Input: dimensioned drawing with shaded views. Units: mm. Origin: part minimum x, y, z. Give positions to 0.01 mm unless a question says otherwise; leave off trailing zeros. Order: outer loops, then holes, each group sorted by start corner. A loop starts at its lowest first (then second) coordinate and runs counter-clockwise, first axis right, second up.
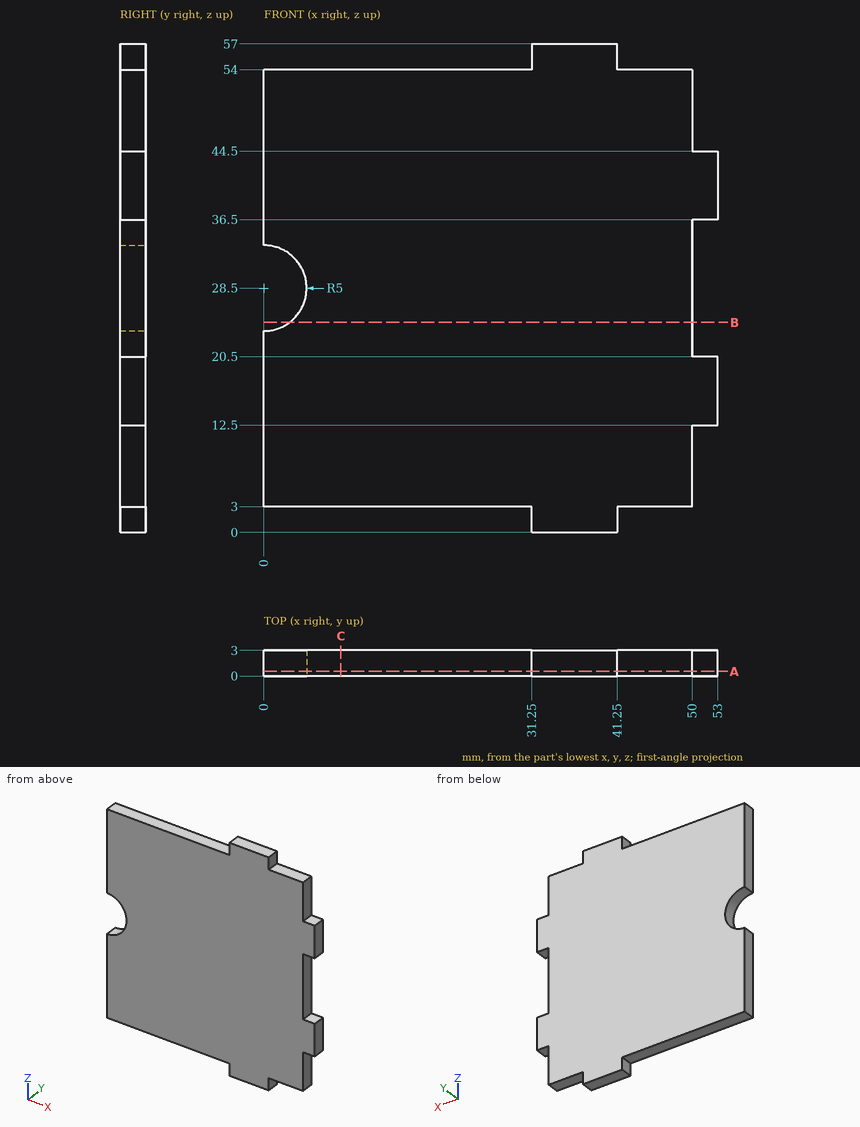
1) Section query B-B, the plane z = 24.5. Return the cut outline in (x, y).
Report:
outline: (3, 0) - (50, 0) - (50, 3) - (3, 3) - close
2) Section query C-C, the plane x = 9. Return the cut outline in (y, z), and give its area (3 significant figures).
Report:
outline: (0, 3) - (3, 3) - (3, 54) - (0, 54) - close
area: 153 mm2
3) Material intervals for L1, parallel to Z at x = 51, y = 0.1; L2, parallel to X at y = 1.2, z = 12; L3, parallel to X at y = 2.5, z = 55, sorted ascending.
Report:
L1: z = 12.5 to 20.5, 36.5 to 44.5
L2: x = 0 to 50
L3: x = 31.25 to 41.25
4) Pin query (flat end, axial travel): pin 1 (0.9 mm diameter, centred on y = 1.5, z = 1, fed in from -X); pin 2 (1.5 mm diameter, centred on x = 46, y = 1.5, fed in from -Z); pin 3 (1.5 mm diameter, centred on x = 24, y = 1, fed in from +Z); pin 4 (1.5 mm diameter, centred on y = 1, z = 35.5, fed in from -X). Return the tip coordinate at first contact, or that it passes through.
Report:
pin 1: stops at x = 31.25
pin 2: stops at z = 3
pin 3: stops at z = 54
pin 4: stops at x = 0
5) Section query A-A, the plane y = 0.55. Return the cut outline in (x, z), and give its area (3 significant figures).
Report:
outline: (0, 3) - (31.25, 3) - (31.25, 0) - (41.25, 0) - (41.25, 3) - (50, 3) - (50, 12.5) - (53, 12.5) - (53, 20.5) - (50, 20.5) - (50, 36.5) - (53, 36.5) - (53, 44.5) - (50, 44.5) - (50, 54) - (41.25, 54) - (41.25, 57) - (31.25, 57) - (31.25, 54) - (0, 54) - (0, 33.5) arc R5 cw to (0, 23.5) - close
area: 2,620 mm2
